The listing builds one solid part. Answer for the finished solid, in the listing's coordinates (mm). A direction names the side the tool comes from. Round coordinates to 2 decimals unless told otherwise and drop trailing zeros. Write each loop counter-clockwise with the first axis right and the second up, starting at its lowest first coordinate (ties: lowest second). Pieces come first, ordered by that corner, then holes. Notation, with made-up numbers: M 44.25,9 L 66.25,9 A27 cw 66.25,27 Z; hole C 87.25,30 d5. An arc over 180 degrees is marked long. Write each question's results on one line, items separated by ' | '.
from build123d import *

# Parameters (mm, degrees)
EXTRUDE_1_DEPTH     = 42
CUT_EXTRUDE_START   = -3
CUT_EXTRUDE_3_DEPTH = 3
CUT_EXTRUDE_4_DEPTH = 3
CUT_EXTRUDE_5_DEPTH = 2


# Read off the part's stored shape, not the designer's step: Вырез-Вытянуть3
with BuildPart() as part:
    # Эскиз1 → Бобышка-Вытянуть1 (new body)
    with BuildSketch(Plane(origin=(0, 0, 0), x_dir=(1, 0, 0), z_dir=(0, 1, 0))):
        with BuildLine():
            Line((-8, -0.75), (8, -0.75))
            Line((8, -0.75), (9.494720433, 0.624258888))
            Line((9.494720433, 0.624258888), (10.065554034, 7.409920575))
            ThreePointArc((10.065554034, 7.409920575), (11.957363782, 9.903499319), (13.236218518, 12.760317415))
            ThreePointArc((13.236218518, 12.760317415), (13.878412353, 16.91337864), (13.236218518, 21.066439864))
            ThreePointArc((13.236218518, 21.066439864), (0.128412353, 30.66337864), (-12.979393813, 21.066439864))
            ThreePointArc((-12.979393813, 21.066439864), (-13.621587647, 16.91337864), (-12.979393813, 12.760317415))
            ThreePointArc((-12.979393813, 12.760317415), (-11.695261173, 9.894600658), (-9.794416407, 7.394977019))
            Line((-9.794416407, 7.394977019), (-9.498544352, 0.683933169))
            Line((-9.498544352, 0.683933169), (-8, -0.75))
        make_face()
        with BuildLine():
            Line((8.578412353, 7.625752463), (8, 0.75))
            Line((8, 0.75), (-8, 0.75))
            Line((-8, 0.75), (-8.321587647, 8.04433134))
            ThreePointArc((-8.321587647, 8.04433134), (-10.262087468, 10.424926322), (-11.549451322, 13.21337864))
            ThreePointArc((-11.549451322, 13.21337864), (-12.121587647, 16.91337864), (-11.549451322, 20.61337864))
            ThreePointArc((-11.549451322, 20.61337864), (0.128412353, 29.16337864), (11.806276027, 20.61337864))
            ThreePointArc((11.806276027, 20.61337864), (12.378412353, 16.91337864), (11.806276027, 13.21337864))
            ThreePointArc((11.806276027, 13.21337864), (10.518912173, 10.424926322), (8.578412353, 8.04433134))
            Line((8.578412353, 8.04433134), (8.578412353, 7.625752463))
        make_face(mode=Mode.SUBTRACT)
    extrude(amount=EXTRUDE_1_DEPTH)

    # Вырез-Вытянуть3 outline → Вырез-Вытянуть3 (cut)
    with BuildSketch(Plane(origin=(0, 42, 0), x_dir=(1, 0, 0), z_dir=(0, 1, 0)).offset(CUT_EXTRUDE_START)):
        with BuildLine():
            Line((-9.498544352, 0.683933169), (-8, -0.75))
            Line((-8, -0.75), (-8, 0.75))
            Line((-8, 0.75), (-8.321587647, 8.04433134))
            ThreePointArc((-8.321587647, 8.04433134), (0.128412353, 29.16337864), (8.578412353, 8.04433134))
            Line((8.578412353, 8.04433134), (8.578412353, 7.625752463))
            Line((8.578412353, 7.625752463), (8, 0.75))
            Line((8, 0.75), (8, -0.75))
            Line((8, -0.75), (9.494720433, 0.624258888))
            Line((9.494720433, 0.624258888), (10.065554034, 7.409920575))
            ThreePointArc((10.065554034, 7.409920575), (0.118066222, 30.663374747), (-9.794416407, 7.394977019))
            Line((-9.794416407, 7.394977019), (-9.498544352, 0.683933169))
        make_face()
    extrude(amount=CUT_EXTRUDE_3_DEPTH, mode=Mode.SUBTRACT)

    # Эскиз5 → Вырез-Вытянуть4 (cut)
    with BuildSketch(Plane.XZ):
        Polygon((-15.223121419, -31.649837006), (15.223121419, -31.649837006), (15.223121419, -0.75), (15.223121419, 0.75), (8, 0.75), (8, -0.75), (-8, -0.75), (-8, 0.75), (-15.223121419, 0.75), (-15.223121419, -0.75), align=None)
    extrude(amount=-CUT_EXTRUDE_4_DEPTH, mode=Mode.SUBTRACT)

    # Эскиз2 → Вырез-Вытянуть5 (cut)
    with BuildSketch(Plane.XY.offset(0.75)):
        Polygon((-6, 3), (-6, 0), (6, 0), (6, 3), (6, 7), (-6, 7), align=None)
        Polygon((-6, 39), (-6, 35), (6, 35), (6, 39), (6, 42), (-6, 42), align=None)
    extrude(amount=-CUT_EXTRUDE_5_DEPTH, mode=Mode.SUBTRACT)


solid = part.part
1) Each of these flat-tipped pins is pushed along its axis until it touches: pin 1 (3 mm diameter, centred on x = -5, y = 19, fed in from -Z); pin 2 (1.6 mm diameter, centred on x = 0.5, z = 0, fed in from -Y); pin 3 (10 mm diameter, centred on x = 5.5, y = 11, fed in from -Z). Where does it stop, or does it pass through?
Return value:
pin 1: z = -30.18 | pin 2: y = 7 | pin 3: z = -30.66
2) Section B-B (y = 37) is taken. Determine the outline of the cut face in (x, z), then the cut area to 3 significant figures.
Return value:
outline: M -9.79,-7.39 A13.75 ccw long 10.07,-7.41 L 9.49,-0.62 L 8,0.75 L 6,0.75 L 6,-0.75 L 8,-0.75 L 8.58,-7.63 L 8.58,-8.04 A12.25 cw long -8.32,-8.04 L -8,-0.75 L -6,-0.75 L -6,0.75 L -8,0.75 L -9.5,-0.68 Z | area: 121 mm²
3) Section D-D (y = 11) is taken. Determine the outline of the cut face in (x, z), then the cut area to 3 significant figures.
Return value:
outline: M -9.79,-7.39 A13.75 ccw long 10.07,-7.41 L 9.49,-0.62 L 8,0.75 L -8,0.75 L -9.5,-0.68 Z; hole M -8.32,-8.04 A12.25 ccw long 8.58,-8.04 L 8.58,-7.63 L 8,-0.75 L -8,-0.75 Z | area: 139 mm²
4) Section A-A (z = -28) is taken. Determine the outline of the cut face in (x, y), then the cut area to 3 significant figures.
Return value:
outline: M -8,3 L -5.08,3 L -5.08,39 L -8,39 Z; M 5.34,3 L 8.26,3 L 8.26,39 L 5.34,39 Z | area: 210 mm²
5) Section C-C (x = -3) is taken. Determine the outline of the cut face in (y, z), then the cut area to 3 significant figures.
Return value:
outline: M 3,-30.3 L 39,-30.3 L 39,-28.76 L 3,-28.76 Z; M 7,-0.75 L 35,-0.75 L 35,0.75 L 7,0.75 Z | area: 97.6 mm²
6) The mould has two halves that part along Z. Classify faces 4 (the face through (-9.65, 20.75, -4.09)), 5 (the face through (-8.16, 20.75, -4.35)), 6 (the face through (0, 7, 0)): +Z half, -Z half, draft (parallel to the pull), parting line (faces both ways), or undercut.
Return value:
face 4: +Z half | face 5: undercut | face 6: draft
7) A tool of negligible diameter and unlimited length cuts with its end or side. For faces 1 (the face through (6, 3, 0)), 2 (the face through (8, 40, 0)), 3 (the face through (-6, 39, 0)), from which of +Z, -Z, +X, -X, +Y, -Y can it reach the whole face along a straight path? Write none if from no direction.
Return value:
face 1: +Z, -Y | face 2: +Z, -Z, +X, +Y | face 3: +Z, +Y
8) Find the intervals of material crossed by line 1 (X direction, y = 14, z = -17); line 2 (Z direction, x = 4.25, y = 16); line 3 (X direction, y = 11.5, z = -15), in increasing order.
Return value:
line 1: -13.62 to -12.12, 12.38 to 13.88 | line 2: -30.03 to -28.45, -0.75 to 0.75 | line 3: -13.49 to -11.97, 12.23 to 13.74
